Check sheet for the modelled part. Datum: model origin and axes. Units: mm. Face numbers are marked on the shaded views. A direction names the side the tool comes from. Round coordinates to 2 decimals unless told otherwise and drop trailing zeros. Loops run counter-clockwise (first coordinate to the right, second up) from the corner with the lowest first, then second, coordinate; pieces in that order, holes last. Notation, with made-up numbers: (87.5, -39.5) -> (115.5, -39.5) arc R33 cw to (115.5, -6.5) -> close; hole circle Ø8 at (7, 62.5). An arc over 180 degrees is marked (long way). Return JSON: item names as keys, results as strings.
from build123d import *

# Parameters (mm, degrees)
SKETCH1_W           = 120
SKETCH1_H           = 75
SKETCH1_R           = 7.5
BOSS_EXTRUDE1_DEPTH = 25
SKETCH2_R           = 12.5
BOSS_EXTRUDE2_DEPTH = 50


with BuildPart() as part:
    # Sketch1 → Boss-Extrude1 (new body)
    with BuildSketch(Plane.XY):
        Rectangle(SKETCH1_W, SKETCH1_H)
        with Locations((35, 21.875)):
            Circle(SKETCH1_R, mode=Mode.SUBTRACT)
        with Locations((-35, 21.875)):
            Circle(SKETCH1_R, mode=Mode.SUBTRACT)
        with Locations((-35, -21.875)):
            Circle(SKETCH1_R, mode=Mode.SUBTRACT)
        with Locations((35, -21.875)):
            Circle(SKETCH1_R, mode=Mode.SUBTRACT)
    extrude(amount=BOSS_EXTRUDE1_DEPTH)

    # Sketch2 → Boss-Extrude2 (add)
    with BuildSketch(Plane.XY.offset(25)):
        Circle(SKETCH2_R)
    extrude(amount=BOSS_EXTRUDE2_DEPTH)


solid = part.part
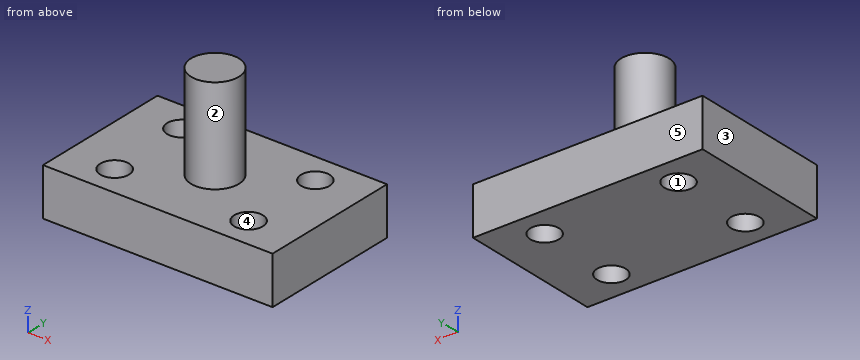
Q1. Draft check along Y on the marked faces 3, 4 and 5. Enter one of: released by +Y, released by -Y, zero draft, split by the parting line, or undercut.
Results list:
{"face 3": "zero draft", "face 4": "undercut", "face 5": "released by +Y"}
Q2. Section check A-A (x = 35). Record the boundary of the cut face in (y, z) (3 decimals).
Results list:
{"outline": "(-37.5, 0) -> (-29.375, 0) -> (-29.375, 25) -> (-37.5, 25) -> close; (-14.375, 0) -> (14.375, 0) -> (14.375, 25) -> (-14.375, 25) -> close; (29.375, 0) -> (37.5, 0) -> (37.5, 25) -> (29.375, 25) -> close"}
Q3. Section check C-C (y = -20.5). Record the boundary of the cut face in (x, z), then the cut area to 3 significant figures.
Results list:
{"outline": "(-60, 0) -> (-42.37, 0) -> (-42.37, 25) -> (-60, 25) -> close; (-27.63, 0) -> (27.63, 0) -> (27.63, 25) -> (-27.63, 25) -> close; (42.37, 0) -> (60, 0) -> (60, 25) -> (42.37, 25) -> close", "area": "2,260 mm^2"}
Q4. Go/stop test with flat-tipped pins: pin 1 (6 mm diameter, centred on y = -2, z = 35.5, fed in from -X); pin 2 (19.5 mm diameter, centred on x = 35, y = -21.875, fed in from +Z). Record where each tip stops, or that it passes through.
Results list:
{"pin 1": "x = -12.5", "pin 2": "z = 25"}
Q5. Section check D-D (z = 12). Record the boundary of the cut face in (x, y) (3 decimals).
Results list:
{"outline": "(-60, -37.5) -> (60, -37.5) -> (60, 37.5) -> (-60, 37.5) -> close; hole circle Ø15 at (-35, -21.875); hole circle Ø15 at (-35, 21.875); hole circle Ø15 at (35, -21.875); hole circle Ø15 at (35, 21.875)"}
Q6. Material ranges on line 1 (Y direction, x = 35, z = 14) (3 decimals); line 2 (X direction, y = -22, z = 5); line 3 (Z direction, x = 53.5, y = 24), recorded low to high.
Results list:
{"line 1": "-37.5 to -29.375, -14.375 to 14.375, 29.375 to 37.5", "line 2": "-60 to -42.5, -27.5 to 27.5, 42.5 to 60", "line 3": "0 to 25"}
Q7. Section check B-B (y = 0). Record the boundary of the cut face in (x, z), then the cut area to 3 significant figures.
Results list:
{"outline": "(-60, 0) -> (60, 0) -> (60, 25) -> (12.5, 25) -> (12.5, 75) -> (-12.5, 75) -> (-12.5, 25) -> (-60, 25) -> close", "area": "4,250 mm^2"}
Q8. Tool access check on the marked faces 1 and 2. Record the directions out of +Z, -Z, +X, -X, +Y, -Y that give a thin tool (end or side, any length) a straight path to the whole face; none if there is none.
Results list:
{"face 1": "+Z, -Z", "face 2": "+Z"}
